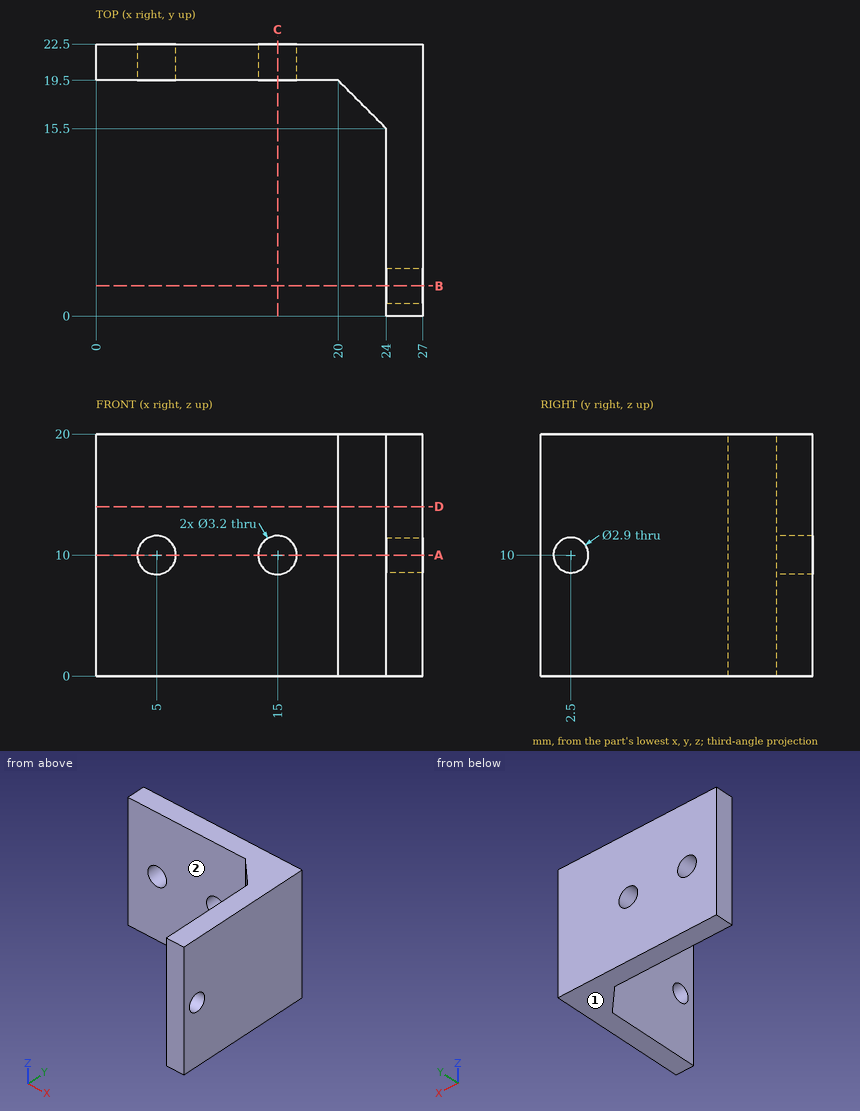
Study the drawing (mm; zero at the part's minimum x, y, z) and answer. A direction names the side the tool comes from. Coordinates: 2 decimals unless noted, no trailing zeros. Write each loop counter-clockwise with the first axis right and the second up, starting at its lowest first coordinate (ties: lowest second). Pieces come first, ordered by that corner, then holes.
Q1. Section B-B, the plane y = 2.5 is taken. Write down the section's boundary in (x, z), then the cut area to 3 significant figures.
Returned:
outline: (24, 0) - (27, 0) - (27, 8.55) - (24, 8.55) - close; (24, 11.45) - (27, 11.45) - (27, 20) - (24, 20) - close
area: 51.3 mm2
Q2. Section C-C, the plane x = 15 is taken. Write down the section's boundary in (y, z), then the cut area to 3 significant figures.
Returned:
outline: (19.5, 0) - (22.5, 0) - (22.5, 8.4) - (19.5, 8.4) - close; (19.5, 11.6) - (22.5, 11.6) - (22.5, 20) - (19.5, 20) - close
area: 50.4 mm2
Q3. Section D-D, the plane z = 14 is taken. Write down the section's boundary in (x, y), then the cut area to 4 significant figures.
Returned:
outline: (0, 19.5) - (20, 19.5) - (24, 15.5) - (24, 0) - (27, 0) - (27, 22.5) - (0, 22.5) - close
area: 147.5 mm2
Q4. Section A-A, the plane z = 10 is taken. Write down the section's boundary in (x, y).
Returned:
outline: (0, 19.5) - (3.4, 19.5) - (3.4, 22.5) - (0, 22.5) - close; (6.6, 19.5) - (13.4, 19.5) - (13.4, 22.5) - (6.6, 22.5) - close; (16.6, 19.5) - (20, 19.5) - (24, 15.5) - (24, 3.95) - (27, 3.95) - (27, 22.5) - (16.6, 22.5) - close; (24, 0) - (27, 0) - (27, 1.05) - (24, 1.05) - close
Q5. Which of the six approach directions +Z, -Z, +X, -X, +Y, -Y give full straight-line access (tool end or side, diameter ignored) to the marked faces 1 and 2?
Returned:
face 1: -Z, +X, -X, +Y, -Y
face 2: +Z, -Z, -X, -Y
Q6. Given P1, Ø2, axis at x = 13, z = 10, coming from the -Y side; P2, Ø4.5, axis at y = 7.5, z = 15, coming from the -X side; P3, Ø1.7, axis at y = 2.5, z = 10, coming from the -X side, each flat-ended and moving along its own axis, determine where each tip first touches the part or whether it passes through.
Returned:
P1: stops at y = 19.5
P2: stops at x = 24
P3: passes through
Q7. Find the intervals of material crossed by line 1 along Y through (x, z) = (25.95, 10); line 2 along Z through (x, y) = (5, 21.45); line 3 along X through (y, z) = (7.75, 9.5), in increasing order.
Returned:
line 1: y = 0 to 1.05, 3.95 to 22.5
line 2: z = 0 to 8.4, 11.6 to 20
line 3: x = 24 to 27
